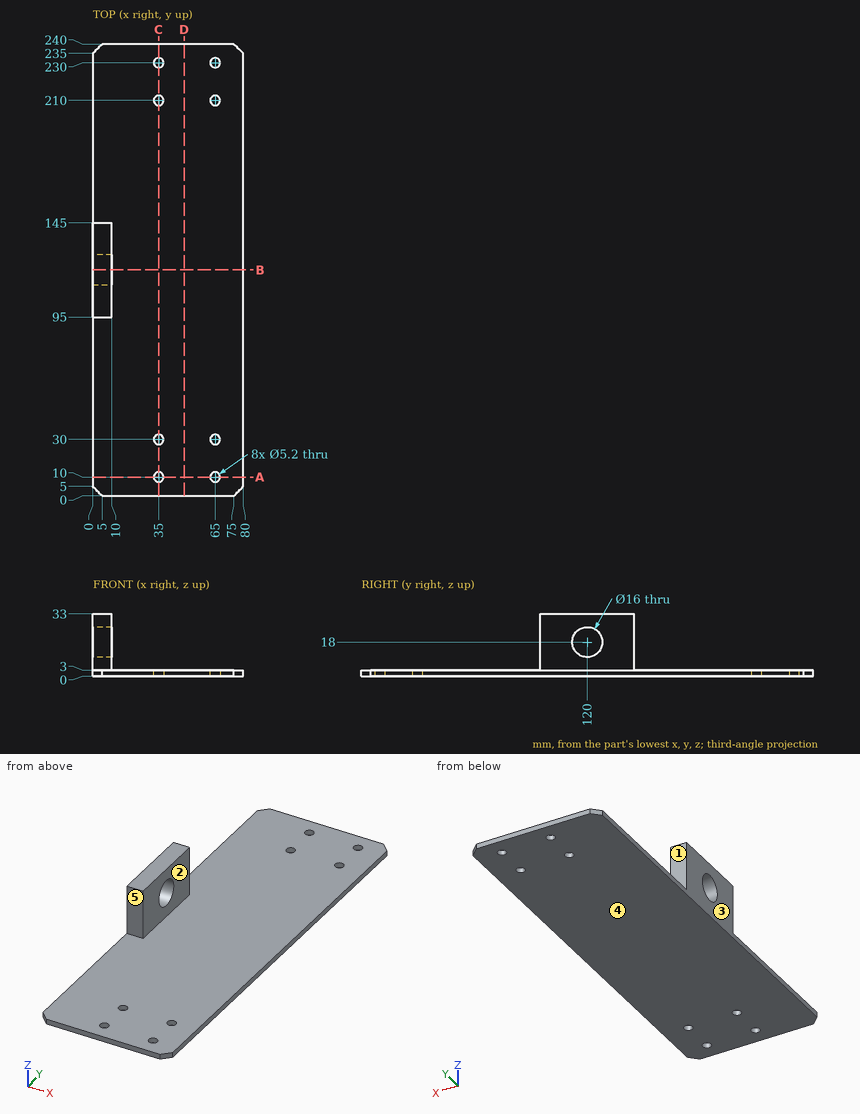
Print and shaded views of the part. All mm, measured from the part's lowest x, y and z. A direction names the side the tool comes from. Round coordinates to 2 decimals unless told otherwise and drop trailing zeros. Order: outer loops, then holes, each group sorted by start corner. A loop starts at its lowest first (then second) coordinate and runs counter-clockwise, first axis right, second up. Notation, with made-up numbers: (26.5, 77.25) - (61.5, 77.25) arc R19 ccw to (61.5, 99.25) - close; hole circle Ø2 at (55.25, 13). An arc over 180 degrees is marked (long way). Use a Markdown table: item, result.
1) Saw through at B-B on y = 120. Write the cut outline in (x, z).
Recorded:
| item | result |
|---|---|
| outline | (0, 0) - (80, 0) - (80, 3) - (10, 3) - (10, 10) - (0, 10) - close; (0, 26) - (10, 26) - (10, 33) - (0, 33) - close |
2) Tool access for the marked faces 1, 2, 3, 4 and 5: list every direction of +Z, -Z, +X, -X, +Y, -Y with a clear straight run to the whole face (end or side of a thin tool).
Recorded:
| item | result |
|---|---|
| face 1 | +Z, +X, -X, +Y |
| face 2 | +Z, +X, +Y, -Y |
| face 3 | +Z, -Z, -X, +Y, -Y |
| face 4 | -Z, +X, -X, +Y, -Y |
| face 5 | +Z, +X, -X, -Y |
3) Saw through at C-C on x = 35. Write the cut outline in (y, z), and give its area (3 significant figures).
Recorded:
| item | result |
|---|---|
| outline | (0, 0) - (7.4, 0) - (7.4, 3) - (0, 3) - close; (12.6, 0) - (27.4, 0) - (27.4, 3) - (12.6, 3) - close; (32.6, 0) - (207.4, 0) - (207.4, 3) - (32.6, 3) - close; (212.6, 0) - (227.4, 0) - (227.4, 3) - (212.6, 3) - close; (232.6, 0) - (240, 0) - (240, 3) - (232.6, 3) - close |
| area | 658 mm² |
4) Wall check: L1, parallel to Y at x = 35, z = 1.8; L2, parallel to X at y = 210, z = 1; L3, parallel to Y at x = 4, z = 5.5. Give the ranges that are in metal, low to high.
Recorded:
| item | result |
|---|---|
| L1 | y = 0 to 7.4, 12.6 to 27.4, 32.6 to 207.4, 212.6 to 227.4, 232.6 to 240 |
| L2 | x = 0 to 32.4, 37.6 to 62.4, 67.6 to 80 |
| L3 | y = 95 to 145 |
5) Flat gauge pins, fed straight in: pin 1 Ø8.5 at (x, y) = (35, 30) entering from -Z; pin 2 Ø7 at (x, y) = (35, 210) entering from +Z; pin 3 Ø8 at (x, z) = (5, 22.5) entering from -Y; pin 4 Ø6 at (y, z) = (95.5, 28) entering from +X. Where does each tip first touch, or does it go through?
Recorded:
| item | result |
|---|---|
| pin 1 | stops at z = 0 |
| pin 2 | stops at z = 3 |
| pin 3 | stops at y = 95 |
| pin 4 | stops at x = 10 |
6) Saw through at D-D on x = 48.5. Write the cut outline in (y, z), and give its area (3 significant figures).
Recorded:
| item | result |
|---|---|
| outline | (0, 0) - (240, 0) - (240, 3) - (0, 3) - close |
| area | 720 mm² |
7) Saw through at A-A on y = 10. Write the cut outline in (x, z).
Recorded:
| item | result |
|---|---|
| outline | (0, 0) - (32.4, 0) - (32.4, 3) - (0, 3) - close; (37.6, 0) - (62.4, 0) - (62.4, 3) - (37.6, 3) - close; (67.6, 0) - (80, 0) - (80, 3) - (67.6, 3) - close |
